Model file for the job. Use its own axes, mm. A direction names the side the tool comes from. Round coordinates to 2 decimals unless told otherwise and drop trailing zeros. Loops run counter-clockwise (first coordinate to the right, second up) from the corner with the lowest first, then second, coordinate; pieces in that order, holes last.
from build123d import *

# Parameters (mm, degrees)
EXTRUDE_339_DEPTH     = 5
SKETCH_D_OUTSIDE_W    = 52.442
SKETCH_D_OUTSIDE_H    = 54.298
SKETCH_D_OUTSIDE_R    = 5.7
CUT_EXTRUDE_383_DEPTH = 10
CUT_EXTRUDE_383_DRAFT = -60
SKETCH_418_R          = 4
EXTRUDE_481_DEPTH     = 20
CHAMFER_526_SIZE      = 1.6


with BuildPart() as part:
    # Sketch 332 → Extrude 339 (new body)
    with BuildSketch(Plane.XY):
        Polygon((0, -6.92820323), (6, -3.464101615), (6, 3.464101615), (0, 6.92820323), (-6, 3.464101615), (-6, -3.464101615), align=None)
    extrude(amount=EXTRUDE_339_DEPTH)


with BuildPart() as cut_extrude_383_tool:
    # D outside → Cut-Extrude 383 (with draft: the straight prism first)
    with BuildSketch(Plane.XY.offset(5)):
        Rectangle(SKETCH_D_OUTSIDE_W, SKETCH_D_OUTSIDE_H)
        Circle(SKETCH_D_OUTSIDE_R, mode=Mode.SUBTRACT)
    extrude(amount=-CUT_EXTRUDE_383_DEPTH)
    # Cut-Extrude 383: the draft: its side faces are tilted about the plane it starts from
    cut_extrude_383_sides = [cut_extrude_383_tool.faces().sort_by_distance(p)[0] for p in [
        (0, -27.149, 0),
        (26.221, 0, 0),
        (0, 27.149, 0),
        (-26.221, 0, 0),
        (-5.7, 0, 0),
    ]]
    draft(cut_extrude_383_sides, Plane.XY.offset(5), CUT_EXTRUDE_383_DRAFT)


with BuildPart() as part_1:
    add(part.part)

    # Cut-Extrude 383: cut by cut_extrude_383_tool
    add(cut_extrude_383_tool.part, mode=Mode.SUBTRACT)

    # Sketch 418 → Extrude 481 (add)
    with BuildSketch(Plane(origin=(0, 0, 0), x_dir=(-1, 0, 0), z_dir=(0, 0, -1))):
        Circle(SKETCH_418_R)
    extrude(amount=EXTRUDE_481_DEPTH)

    # Chamfer 526
    chamfer_526_edges = [part_1.edges().sort_by_distance(p)[0] for p in [
        (4, 0, -20),
    ]]
    chamfer(chamfer_526_edges, length=CHAMFER_526_SIZE)


solid = part_1.part
Q1. Slice it at A-A on y = 0. Give the cut face in (x, z), plus the area to 3 significant figures.
Q2. Probe line 1 (Z direction, x = 3.5, y = -3.5); line 2 (Z direction, x = -0.75, y = -2.5); line 3 (Y direction, x = -2.5, z = -8). List the from-to ranges inside material, lowest first.
Q3. Flat gauge pins, fed straight in: P1, Ø6, axis at x = 3, z = -4.5, coming from the +Y side; P2, Ø5, axis at y = -0.5, z = -16, coming from the +X side; P3, Ø2, axis at y = -3.5, z = -6.5, coming from the +X side. Where does each tip first touch, or does it go through?
Q4. Tool access for faces 1 (the face through (-3, -3, 0)), 2 (the face through (0, 0, -20)): list every direction of +Z, -Z, +X, -X, +Y, -Y with a clear straight run to the whole face (end or side of a thin tool).
Q5. Slice it at C-C on z = -8.25. Give the cut face in (x, y).
Q6. Slice it at B-B on z = 0.25. Give the cut face in (x, y), plus the area to 3 significant figures.
Reply:
1. outline: (-6, 0) - (-4, 0) - (-4, -18.4) - (-2.4, -20) - (2.4, -20) - (4, -18.4) - (4, 0) - (6, 0) - (6, 4.83) - (5.7, 5) - (-5.7, 5) - (-6, 4.83) - close
1. area: 217 mm2
2. line 1: z = 0 to 5
2. line 2: z = -19.79 to 5
2. line 3: y = -3.12 to 3.12
3. P1: stops at y = 4
3. P2: stops at x = 4
3. P3: stops at x = 3.12
4. face 1: -Z
4. face 2: -Z, +X, -X, +Y, -Y
5. outline: circle Ø8 at (0, 0)
6. outline: (-6, -3.46) - (0, -6.93) - (6, -3.46) - (6, 3.46) - (0, 6.93) - (-6, 3.46) - close
6. area: 125 mm2
